```python
from build123d import *

# Parameters (mm, degrees)
F1_DEPTH      = 1981.2
F3_W          = 96.8375
F3_H          = 12.7
F4_DEPTH      = 76.2
F4_DEPTH_BACK = 76.2
F5_W          = 101.6
F5_H          = 9.525
F6_DEPTH      = 1041.4
F6_DEPTH_BACK = 1041.4
F7_W          = 50.8
F7_H          = 19.05
F7_W_2        = 38.099998
F8_DEPTH      = 1041.4
F8_DEPTH_BACK = 1041.4


with BuildPart() as f1:
    # F0 (on Top) → F1 (new body)
    with BuildSketch(Plane.XY):
        Polygon((-48.41875, -50.8), (-48.41875, 0), (-53.18125, 0), (-53.18125, -51.514181), (-30.507902, -125.4125), (30.507902, -125.4125), (53.18125, -51.514181), (53.18125, 0), (48.41875, 0), (48.41875, -50.8), (26.9875, -120.65), (-26.9875, -120.65), align=None)
    extrude(amount=F1_DEPTH)

    # F3 (on offset) → F4 (join, two sides)
    with BuildSketch(Plane.XY.offset(990.6)) as f4_sk:
        with Locations((0, -6.35)):
            Rectangle(F3_W, F3_H)
    extrude(amount=F4_DEPTH)
    extrude(f4_sk.sketch, amount=-F4_DEPTH_BACK)

    # F5 (on offset) → F6 (join, two sides)
    with BuildSketch(Plane.XY.offset(990.6)) as f6_sk:
        with Locations((0, 4.7625)):
            Rectangle(F5_W, F5_H)
    extrude(amount=F6_DEPTH)
    extrude(f6_sk.sketch, amount=-F6_DEPTH_BACK)

    # F7 (on offset) → F8 (join, two sides)
    with BuildSketch(Plane.XY.offset(990.6)) as f8_sk:
        with Locations((48.418748, 19.05)):
            Rectangle(F7_W, F7_H)
        with Locations((-46.831251, 19.05)):
            Rectangle(F7_W_2, F7_H)
    extrude(amount=F8_DEPTH)
    extrude(f8_sk.sketch, amount=-F8_DEPTH_BACK)


solid = f1.part
```
Part model, mm, in its own coordinate system. A direction names the side the tool comes from. Give positions to 0.01 mm unless a question says otherwise; leave off trailing zeros. Loops run counter-clockwise (first coordinate to the right, second up) from the corner with the lowest first, then second, coordinate; pieces in that order, holes last. Notation, with made-up numbers: M 3.25,61 L 55.25,61 A13 ccw 55.25,73 Z; hole C 85.25,79.5 d11. An arc over 180 degrees is marked long. Return JSON: item names as keys, results as strings.
1) Pull direction X, two halves, no side cores. Call faces 1 (the face through (-53.181, -25, 977)), 2 (the face through (48, 28.575, 1005)), 3 (the face through (53.181, -26, 977)), 4 (the face through (-1, 0, 439)): released by +X, released by -X, zero draft, split by the parting line, or undercut.
Calculated:
{"face 1": "released by -X", "face 2": "zero draft", "face 3": "released by +X", "face 4": "undercut"}
2) 3-axis set-ups, long thin cutter, end or side, ignore diameter. For faces 5 (the face through (-3, 9.525, 1005)), 6 (the face through (-1, 0, 1543)), 7 (the face through (0, -120.65, 977)): which of +Z, -Z, +X, -X, +Y, -Y reach the whole face in a straight line?
Calculated:
{"face 5": "+Z, -Z, +Y", "face 6": "+Z", "face 7": "+Z, -Z"}
3) Saw through at B-B, the plane y = -69. List the corners of the cut face in (x, z).
Calculated:
{"outline": "M -47.82,0 L -42.83,0 L -42.83,1981.2 L -47.82,1981.2 Z; M 42.83,0 L 47.82,0 L 47.82,1981.2 L 42.83,1981.2 Z"}
4) Drill centre lines: line 1 (X direction, y = -52, z = 351); line 2 (Y direction, x = 63, z = 244.5) (3 decimals); line 3 (Z direction, x = 52, y = -23). Where is each one in solid material? Low to high.
Calculated:
{"line 1": "x = -53.03 to -48.05, 48.05 to 53.03", "line 2": "y = 9.525 to 28.575", "line 3": "z = 0 to 1981.2"}
5) Flat gauge pins, fed straight in: pin 1 Ø2 at (x, z) = (-17, 1751.5) entering from +Y (3 decimals); pin 2 Ø1 at (y, z) = (-73, 860.5) entering from +X; pin 3 Ø2 at (y, z) = (-103.5, 788) entering from +X. Where does each tip first touch, or does it go through?
Calculated:
{"pin 1": "stops at y = 9.525", "pin 2": "stops at x = 46.74", "pin 3": "stops at x = 37.54"}
